Could you check a few things on this model? Use its own coordinates, in mm. Round coordinates to 2 decimals unless told otherwise and drop trailing zeros. Order: outer loops, then holes, each group sorted by start corner. A loop starts at its lowest first (then second) coordinate and runs counter-clockwise, first axis right, second up.
Autodesk Inventor part; units mm, degrees
ref_plane "YZ Plane" through (0, 0, 0) normal (1, 0, 0) x (0, 1, 0)
ref_plane "XZ Plane" through (0, 0, 0) normal (0, 1, 0) x (-1, 0, 0)
ref_plane "XY Plane" through (0, 0, 0) normal (0, 0, 1) x (1, 0, 0)
sketch "Sketch1" plane through (0, 0, 0) normal (0, 0, 1) x (1, 0, 0)
  line L0 (12.7, 0) -> (12.7, 12.7)
  circle A0 centre (-76, -52) radius 1.4224
  line L1 (-88.7, -64.7) -> (-76, -64.7)
  line L2 (-88.7, -64.7) -> (12.7, -64.7)
  line L3 (12.7, -64.7) -> (12.7, 12.7)
  line L4 (12.7, 12.7) -> (-88.7, 12.7)
  line L5 (-88.7, 12.7) -> (-88.7, -64.7)
  line L6 (-88.7, 12.7) -> (-76, 12.7)
  line L7 (-88.7, 0) -> (-88.7, 12.7)
  line L8 (-88.7, -64.7) -> (-76, -64.7)
  line L9 (-88.7, -52) -> (-88.7, -64.7)
  line L10 (12.7, -64.7) -> (0, -64.7)
  line L11 (12.7, 12.7) -> (0, 12.7)
  line L12 (12.7, 0) -> (12.7, 12.7)
  circle A1 centre (-76, 0) radius 1.1049
  circle A2 centre (-76, -52) radius 1.1049
  circle A3 centre (0, 0) radius 1.1049
  circle A4 centre (0, -52) radius 1.1049
  dimension "d1" = 12.7
  dimension "d2" = 12.7
  dimension "d10" = 12.7
  dimension "d11" = 12.7
  dimension "d12" = 2.2098
  dimension "d13" = 2.2098
  dimension "d14" = 2.2098
  dimension "d15" = 2.2098
extrude "Extrusion2" add sketch "Sketch1" against normal blind 2.54 contours L3 L2 L1 L5 L4 L0
properties part number "BasePlate"
Q1. Imagine slicing it at B-B, the plane x = -76. Please give me the cut outline in (y, z).
Q2. We'd pull the mould along Y, two halves only. Please class faces 1 (the flat face through (-37, 12.7, -1)), 2 (the cylindrical face through (-0.1, 1.1, -1.3)), 3 (the flat face through (-39, -25, 0)): released by +Y, released by -Y, zero draft, split by the parting line, or undercut.
Q3. Imagine slicing it at A-A, the plane y = -52. Please give me the cut outline in (x, z).
Q4. I need wall thicknesses on L1, parallel to Y at x = -76, z = -0.55; L2, parallel to Y at x = 0, z = -1.25. Which ranges of each line are inside material? Lowest first, please.
Q5. For P1, Ø2, axis at x = 0, y = 0, coming from the +Z side, with a flat end and sliding along its axis, tell me the tip position at first contact or that it passes through.
Filled in:
1. outline: (-64.7, -2.54) - (-53.42, -2.54) - (-53.42, 0) - (-64.7, 0) - close; (-50.58, -2.54) - (-1.1, -2.54) - (-1.1, 0) - (-50.58, 0) - close; (1.1, -2.54) - (12.7, -2.54) - (12.7, 0) - (1.1, 0) - close
2. face 1: released by +Y
2. face 2: undercut
2. face 3: zero draft
3. outline: (-88.7, -2.54) - (-77.42, -2.54) - (-77.42, 0) - (-88.7, 0) - close; (-74.58, -2.54) - (-1.1, -2.54) - (-1.1, 0) - (-74.58, 0) - close; (1.1, -2.54) - (12.7, -2.54) - (12.7, 0) - (1.1, 0) - close
4. L1: y = -64.7 to -53.42, -50.58 to -1.1, 1.1 to 12.7
4. L2: y = -64.7 to -53.1, -50.9 to -1.1, 1.1 to 12.7
5. P1: passes through
